Autodesk Fusion 360 part; units mm, degrees
sketch "Sketch2" plane through (0, 0, 0) normal (0, 0, 1) x (1, 0, 0)
  line L0 (25, -15) -> (-25, -15)
  line L1 (-25, -15) -> (-25, 15)
  line L2 (-25, 15) -> (25, 15)
  line L3 (25, 15) -> (25, -15)
  line L4 (25, -15) -> (-25, 15) construction
  line L5 (-25, -15) -> (25, 15) construction
  dimension "d3" = 50
  dimension "d4" = 30
extrude "Extrude1" add sketch "Sketch2" along normal blind 2
sketch "Sketch3" plane through (0, 0, 2) normal (0, 0, 1) x (-1, 0, 0)
  line L0 (-25, -15) -> (25, -15)
  line L1 (25, -15) -> (25, 15)
  line L2 (25, 15) -> (-25, 15)
  line L3 (-25, 15) -> (-25, -15)
  circle A0 centre (9, 0) radius 8.875
  circle A1 centre (9, 0) radius 12
  dimension "d7" = 17.75
  dimension "d8" = 24
  dimension "d9" = 16
extrude "Extrude2" cut sketch "Sketch3" against normal blind 4 contours A0
sketch "Sketch4" plane through (0, 0, 0) normal (0, 0, -1) x (1, 0, 0)
  circle A0 centre (-9, 0) radius 8.875
  line L0 (-25, -15) -> (25, -15)
  line L1 (25, -15) -> (25, 15)
  line L2 (25, 15) -> (-25, 15)
  line L3 (-25, 15) -> (-25, -15)
  line L4 (25, 15) -> (11, 15)
  line L5 (11, 15) -> (11, -15)
  line L6 (11, -15) -> (25, -15)
  line L7 (25, -15) -> (25, 15)
  dimension "d12" = 14
extrude "Extrude3" add sketch "Sketch4" along normal blind 7 contours L0 L1 L2 L4 L5 L6 L7
fillet "Fillet1" radius 2 1 edges at (11, 0, 0)
fillet "Fillet2" radius 2 1 edges at (-0.7256, 3.2093, 0)
sketch "Sketch5" plane through (0, 0, -7) normal (0, 0, -1) x (1, 0, 0)
  line L0 (25, -15) -> (25, 15)
  line L1 (25, 15) -> (11, 15)
  line L2 (11, 15) -> (11, -15)
  line L3 (11, -15) -> (25, -15)
  line L4 (15, 11) -> (21, 11)
  line L5 (21, 11) -> (21, -11)
  line L6 (21, -11) -> (15, -11)
  line L7 (15, -11) -> (15, 11)
  dimension "d19" = 4
  dimension "d20" = 4
  dimension "d21" = 4
  dimension "d22" = 4
extrude "Extrude4" cut sketch "Sketch5" against normal blind 17 contours L4 L5 L6 L7
equation "d20 = d19"
equation "d21 = d19"
equation "d22 = d19"
Input: part model. Units: mm. Frame: model coordinates. A direction names the side the tool comes from. Give positions to 0.01 mm unless a question says otherwise; leave off trailing zeros. Loops run counter-clockwise (first coordinate to the right, second up) from the corner with the lowest first, then second, coordinate; pieces in that order, holes last. Notation, with made-up numbers: (-24, 61.25) -> (21, 61.25) arc R19 cw to (21, 80.25) -> close; hole circle Ø8 at (-11.5, 66). An arc over 180 degrees is marked (long way). Answer as a JSON object with one key per item and string values. Group by question number.
Item 1: Cut plane A-A, the plane z = -3.25. Return the cut outline in (x, y), and give its area (3 significant figures).
Item 2: Cut plane D-D, the plane z = 1.5. Return the cut outline in (x, y).
Item 3: Reachability of faces 1 (the flat face through (25, 0, -2)), 2 (the flat face through (-4, 10, 0)), 3 (the flat face through (15, 0, -3)) from +Z, -Z, +X, -X, +Y, -Y: full face, straight path, thin tool, end or side. Return the list, or none.
Item 4: Line query: probe 1 along X at (y, z) = (-8.5, -2.5); probe 2 along Y at (x, z) = (16, -6); probe 3 along Z at (x, y) = (-4.5, 10.5). Output: solid intervals per line, ascending.
Item 5: Pin query (flat end, axial travel): P1, Ø1.5, axis at y = 3.5, z = -3.5, coming from the -X side; P2, Ø15, axis at x = -7.5, y = -5, coming from the -Z side. Return the tip coordinate at first contact, or that it passes through.
Item 6: Cut plane C-C, the plane y = 0. State how many separate pieces and enclosed holes the cut face has, and give its area (3 significant figures).
Checks:
{
 "1": {"outline": "(11, -15) -> (25, -15) -> (25, 15) -> (11, 15) -> close; hole (15, -11) -> (21, -11) -> (21, 11) -> (15, 11) -> close", "area": "288 mm²"},
 "2": {"outline": "(-25, -15) -> (25, -15) -> (25, 15) -> (-25, 15) -> close; hole circle Ø17.88 at (-9, 0); hole (15, -11) -> (21, -11) -> (21, 11) -> (15, 11) -> close"},
 "3": {"face 1": "+Z, -Z, +X, +Y, -Y", "face 2": "-Z, -X, +Y, -Y", "face 3": "+Z, -Z"},
 "4": {"probe 1": "x = 11 to 15, 21 to 25", "probe 2": "y = -15 to -11, 11 to 15", "probe 3": "z = 0 to 2"},
 "5": {"P1": "stops at x = 11", "P2": "stops at z = 0"},
 "6": {"separate pieces": "3", "enclosed holes": "0", "area": "108 mm²"}
}
